```python
from build123d import *

# Parameters (mm, degrees)
ESBO_O1_R                = 20
ESBO_O1_R_2              = 2.85
ESBO_O1_R_3              = 2
ESBO_O1_R_4              = 1.6
RESSALTO_EXTRUS_O1_DEPTH = 3


with BuildPart() as part:
    # Esboço1 → Ressalto-extrusão1 (new body)
    with BuildSketch(Plane.XZ.offset(3)):
        Circle(ESBO_O1_R)
        Circle(ESBO_O1_R_2, mode=Mode.SUBTRACT)
        with Locations((10.557104243, 10.557104243)):
            Circle(ESBO_O1_R_3, mode=Mode.SUBTRACT)
        with Locations((10.557104243, -10.557104243)):
            Circle(ESBO_O1_R_3, mode=Mode.SUBTRACT)
        with Locations((-10.557104243, -10.557104243)):
            Circle(ESBO_O1_R_3, mode=Mode.SUBTRACT)
        with Locations((-10.557104243, 10.557104243)):
            Circle(ESBO_O1_R_3, mode=Mode.SUBTRACT)
        with Locations((-8, 0)):
            Circle(ESBO_O1_R_4, mode=Mode.SUBTRACT)
        with Locations((-4, 6.92820323)):
            Circle(ESBO_O1_R_4, mode=Mode.SUBTRACT)
        with Locations((4, 6.92820323)):
            Circle(ESBO_O1_R_4, mode=Mode.SUBTRACT)
        with Locations((8, 0)):
            Circle(ESBO_O1_R_4, mode=Mode.SUBTRACT)
        with Locations((4, -6.92820323)):
            Circle(ESBO_O1_R_4, mode=Mode.SUBTRACT)
        with Locations((-4, -6.92820323)):
            Circle(ESBO_O1_R_4, mode=Mode.SUBTRACT)
    extrude(amount=-RESSALTO_EXTRUS_O1_DEPTH)


solid = part.part
```
For this review, take the finished solid that the model builds, in its own axes (mm). Round coordinates to 2 decimals unless told otherwise and drop trailing zeros. Write each loop counter-clockwise with the first axis right and the second up, starting at its lowest first coordinate (ties: lowest second). Pieces come first, ordered by that corner, then holes. Notation, with made-up numbers: (5, 19.5) - (20, 19.5) arc R21 ccw to (20, 54.5) - close; hole circle Ø8 at (15, -16.75). An arc over 180 degrees is marked (long way). Put each result on its own line as item: value.
Q1. Wall thickness on probe 1 along Z at (x, y) = (0, -2.65); probe 2 along Z at (x, y) = (4, -1.75); probe 3 along X at (y, z) = (-2.7, -8): over which ranges is each line inside the solid? List them lowest first.
Solved:
probe 1: z = -20 to -2.85, 2.85 to 20
probe 2: z = -19.6 to -8.53, -5.33 to 5.33, 8.53 to 19.6
probe 3: x = -18.33 to -5.19, -2.81 to 2.81, 5.19 to 18.33
Q2. We need section C-C (x = 4). Give the boundary of the cut face in (y, z), and give its area (3 significant figures).
Solved:
outline: (-3, -19.6) - (0, -19.6) - (0, -8.53) - (-3, -8.53) - close; (-3, -5.33) - (0, -5.33) - (0, 5.33) - (-3, 5.33) - close; (-3, 8.53) - (0, 8.53) - (0, 19.6) - (-3, 19.6) - close
area: 98.4 mm2
Q3. Mouldability with a two-part tool opening along Z and no side actions: class faces 1 (the face through (-4.336, -1.521, -19.524)), 2 (the face through (0, -3, -4)), 3 (the face through (3.653, -1.521, 5.366)), 4 (the face through (10.12, -1.52, -12.51)) as released by +Z, released by -Z, zero draft, split by the parting line, or undercut.
Solved:
face 1: split by the parting line
face 2: zero draft
face 3: undercut
face 4: undercut
Q4. We need section D-D (z = -7.5). Give the boundary of the cut face in (x, y), and give its area (3 significant figures).
Solved:
outline: (-18.54, -3) - (-5.49, -3) - (-5.49, 0) - (-18.54, 0) - close; (-2.51, -3) - (2.51, -3) - (2.51, 0) - (-2.51, 0) - close; (5.49, -3) - (18.54, -3) - (18.54, 0) - (5.49, 0) - close
area: 93.3 mm2
Q5. We need section A-A (z = 0). Give the boundary of the cut face in (x, y).
Solved:
outline: (-20, -3) - (-9.6, -3) - (-9.6, 0) - (-20, 0) - close; (-6.4, -3) - (-2.85, -3) - (-2.85, 0) - (-6.4, 0) - close; (2.85, -3) - (6.4, -3) - (6.4, 0) - (2.85, 0) - close; (9.6, -3) - (20, -3) - (20, 0) - (9.6, 0) - close
Q6. We need section B-B (x = 0). Give the boundary of the cut face in (y, z), and give its area (3 significant figures).
Solved:
outline: (-3, -20) - (0, -20) - (0, -2.85) - (-3, -2.85) - close; (-3, 2.85) - (0, 2.85) - (0, 20) - (-3, 20) - close
area: 103 mm2
